Can you work these out from the model? Positions are in its coordinate system, mm. A direction names the side the tool comes from. Coordinates: 2 decimals unless noted, no trailing zeros. Loops run counter-clockwise (first coordinate to the right, second up) from the corner with the lowest first, then second, coordinate; pieces in that order, holes last. Notation, with made-up numbers: M 15.5,44.25 L 49.5,44.25 A14 ccw 49.5,60.25 Z; hole C -9.5,-14.5 d10. An arc over 180 degrees is marked long. Answer as a JSON object with one key per item and string values. Group by question number.
Item 1: Which directions (+Z, -Z, +X, -X, +Y, -Y) give clear straight access to the entire face, cutting with the end or side of a thin tool? Please do faces 1 (the flat face through (-32.179, 2, 9)), 2 (the flat face through (3, 2, -13.659)), 3 (the flat face through (50, 2, 1.341)).
Item 2: Suppose I cut it at A-A (y = 2.3). Write out the boundary of the cut face in (x, z).
Item 3: Suppose I cut it at B-B (z = 5.5). Write out the boundary of the cut face in (x, y).
Item 4: If I drill on line 1 (X direction, y = 2.7, z = 12); line 2 (X direction, y = 0.35, z = 6.25), over which ranges is the centre line in solid material (lowest first)?
Item 5: Suppose I cut it at C-C (x = -34.5). Write out the boundary of the cut face in (y, z), then the cut area to 3 significant figures.
Item 6: I'm going to push flat-ended pins straight in: pin 1 Ø1 at (y, z) = (1.5, 9) entering from -X; pin 2 Ø5 at (x, z) = (28.82, 11.34) entering from -Y; pin 3 Ø2.5 at (x, z) = (-21.18, 11.34) entering from -Y; pin 4 Ø1.2 at (y, z) = (3, 12) entering from +X. Where does each tip first touch, or does it pass through?
Item 7: We'd pull the mould along Z, two halves only. Please class faces 4 (the flat face through (-42, 2, 1.341)), 5 (the cylindrical face through (27.323, 2.028, 11.275)), 6 (the flat face through (39.821, 2, 9)): +Z half, -Z half, draft (parallel to the pull), parting line (faces both ways), or undercut.
```python
from build123d import *

# Parameters (mm, degrees)
SKETCH1_W           = 72
SKETCH1_H           = 30
BOSS_EXTRUDE1_DEPTH = 4
SKETCH2_R           = 1.5
CUT_EXTRUDE1_DEPTH  = 4
SKETCH3_W           = 20
SKETCH3_H           = 15
BOSS_EXTRUDE3_DEPTH = 4


with BuildPart() as part:
    # Sketch1 → Boss-Extrude1 (new body)
    with BuildSketch(Plane(origin=(0, 0, 0), x_dir=(1, 0, 0), z_dir=(0, 1, 0))):
        with Locations((3.82122905, -1.340782123)):
            Rectangle(SKETCH1_W, SKETCH1_H)
    extrude(amount=BOSS_EXTRUDE1_DEPTH)

    # Sketch2 → Cut-Extrude1 (cut)
    with BuildSketch(Plane(origin=(0, 4, 0), x_dir=(1, 0, 0), z_dir=(0, 1, 0))):
        with Locations((-21.17877095, -11.340782123)):
            Circle(SKETCH2_R)
        with Locations((28.82122905, -11.340782123)):
            Circle(SKETCH2_R)
    extrude(amount=-CUT_EXTRUDE1_DEPTH, mode=Mode.SUBTRACT)

    # Sketch3 → Boss-Extrude3 (add)
    with BuildSketch(Plane(origin=(0, 4, 0), x_dir=(1, 0, 0), z_dir=(0, 1, 0))):
        with Locations((49.82122905, 6.159217877)):
            Rectangle(SKETCH3_W, SKETCH3_H)
        with Locations((-42.17877095, 6.159217877)):
            Rectangle(SKETCH3_W, SKETCH3_H)
    extrude(amount=-BOSS_EXTRUDE3_DEPTH)


solid = part.part
```
From the geometry:
{
 "1": {"face 1": "+Z, -X, +Y, -Y", "face 2": "-Z, +X, -X, +Y, -Y", "face 3": "+Z, +X, +Y, -Y"},
 "2": {"outline": "M -52.18,-13.66 L 59.82,-13.66 L 59.82,1.34 L 39.82,1.34 L 39.82,16.34 L -32.18,16.34 L -32.18,1.34 L -52.18,1.34 Z; hole C -21.18,11.34 d3; hole C 28.82,11.34 d3"},
 "3": {"outline": "M -32.18,0 L 39.82,0 L 39.82,4 L -32.18,4 Z"},
 "4": {"line 1": "-32.18 to -22.53, -19.83 to 27.47, 30.17 to 39.82", "line 2": "-32.18 to 39.82"},
 "5": {"outline": "M 0,-13.66 L 4,-13.66 L 4,1.34 L 0,1.34 Z", "area": "60.0 mm2"},
 "6": {"pin 1": "x = -32.18", "pin 2": "y = 0", "pin 3": "through", "pin 4": "x = 39.82"},
 "7": {"face 4": "+Z half", "face 5": "undercut", "face 6": "draft"}
}
